from build123d import *

# Parameters (mm, degrees)
PAD_DEPTH       = 4.5
PAD001_DEPTH    = 140
SKETCH002_R     = 20
PAD002_DEPTH    = 17
SKETCH003_R     = 15.5
POCKET_DEPTH    = 17
POCKET001_DEPTH = 140
FILLET_R        = 2
CHAMFER_SIZE    = 2
SKETCH005_R     = 4.5
SKETCH005_R_2   = 1.45
POCKET002_DEPTH = 5


with BuildPart() as part:
    # Sketch → Pad (new body)
    with BuildSketch(Plane.XZ):
        with BuildLine():
            ThreePointArc((14.282857, 14), (-20, 0), (14.282857, -14))
            Line((14.282857, -14), (125.717143, -14))
            ThreePointArc((125.717143, -14), (160, 0), (125.717143, 14))
            Line((14.282857, 14), (125.717143, 14))
        make_face()
    extrude(amount=PAD_DEPTH)

    # Sketch001 → Pad001 (join)
    with BuildSketch(Plane.YZ):
        Polygon((0, 8.637), (10.293176, 0), (0, -8.637), (0, -14), (16.68455, 0), (0, 14), align=None)
    extrude(amount=PAD001_DEPTH)

    # Sketch002 (on Face4 of Pad001) → Pad002 (join)
    with BuildSketch(Plane(origin=(0, 0, 0), x_dir=(1, 0, 0), z_dir=(0, 1, 0))):
        Circle(SKETCH002_R)
        with Locations((140, 0)):
            Circle(SKETCH002_R)
    extrude(amount=PAD002_DEPTH)

    # Sketch003 (on Face9 of Pad002) → Pocket (cut)
    with BuildSketch(Plane(origin=(0, 17, 0), x_dir=(1, 0, 0), z_dir=(0, 1, 0))):
        Circle(SKETCH003_R)
        with Locations((140, 0)):
            Circle(SKETCH003_R)
    extrude(amount=-POCKET_DEPTH, mode=Mode.SUBTRACT)

    # Sketch004 → Pocket001 (cut)
    with BuildSketch(Plane.YZ):
        Polygon((0, 8.635), (0, -8.635), (10.290792, 0), align=None)
    extrude(amount=POCKET001_DEPTH, mode=Mode.SUBTRACT)

    # Fillet
    fillet_edges = [part.edges().sort_by_distance(p)[0] for p in [
        (120, 17, 0),
        (124.5, 17, 0),
        (-20, 17, 0),
        (-15.5, 17, 0),
    ]]
    fillet(fillet_edges, radius=FILLET_R)

    # Chamfer
    chamfer_edges = [part.edges().sort_by_distance(p)[0] for p in [
        (-20, -4.5, 0),
        (70, -4.5, -14),
        (160, -4.5, 0),
        (70, -4.5, 14),
    ]]
    chamfer(chamfer_edges, length=CHAMFER_SIZE)

    # Sketch005 (on Face29 of Chamfer) → Pocket002 (cut)
    with BuildSketch(Plane(origin=(0, 0, 0), x_dir=(1, 0, 0), z_dir=(0, 1, 0))):
        Circle(SKETCH005_R)
        with Locations((13, 0)):
            Circle(SKETCH005_R_2)
        with Locations((-13, 0)):
            Circle(SKETCH005_R_2)
        with Locations((140, 0)):
            Circle(SKETCH005_R)
        with Locations((153, 0)):
            Circle(SKETCH005_R_2)
        with Locations((127, 0)):
            Circle(SKETCH005_R_2)
        with Locations((0, 13)):
            Circle(SKETCH005_R_2)
        with Locations((0, -13)):
            Circle(SKETCH005_R_2)
        with Locations((140, 13)):
            Circle(SKETCH005_R_2)
        with Locations((140, -13)):
            Circle(SKETCH005_R_2)
    extrude(amount=-POCKET002_DEPTH, mode=Mode.SUBTRACT)


solid = part.part
Could you check a few things on this model? Use its own coordinates, in mm. A direction names the side the tool comes from. Give positions to 0.01 mm unless a question says otherwise; leave off trailing zeros. Loops run counter-clockwise (first coordinate to the right, second up) from the corner with the lowest first, then second, coordinate; pieces in that order, holes last. Notation, with made-up numbers: M 53.5,23.5 L 69.5,23.5 A27 cw 69.5,51.5 Z; hole C 72.25,39.25 d9. An arc over 180 degrees is marked long. Answer as a JSON object with one key per item and string values.
Q1. For faces 3 (the cylindrical face through (141.339, -2.218, -12.445)), 4 (the cylindrical face through (-15.485, 7.605, -0.682)), 5 (the flat face through (17.18, 5.07, -4.38)), which set-ups out of +Z, -Z, +X, -X, +Y, -Y let a thin tool reach every point of the face, with its end or its side?
Values found:
{"face 3": "+Y, -Y", "face 4": "+Y", "face 5": "none"}
Q2. If I drill on probe 1 along X at (y, z) = (7, 0); probe 2 along X at (y, z) = (14.5, 13); probe 3 along X at (y, z) = (-3.45, -13), over which ranges is the centre line in solid material (lowest first)? Write a range as [from, to].
Values found:
{"probe 1": "x = [-20, -15.5], [155.5, 160]", "probe 2": "x = [-15.2, -8.44], [8.44, 15.2], [124.8, 131.56], [148.44, 155.2]", "probe 3": "x = [-13.92, -1.45], [1.45, 138.55], [141.45, 153.92]"}
Q3. If we mould it in two halves opening along X, with no side actions, what happens to faces 1 (the flat face through (69, -4.5, 0)), 2 (the cylindrical face through (154.318, 7.605, 5.937))? For each: pulls with the +X half, pulls with the -X half, needs draft (parallel to the pull), parting line crosses it, or undercut.
Values found:
{"face 1": "needs draft", "face 2": "undercut"}
Q4. Suppose I cut it at A-A, the plane x = 37. List the corners of the cut face in (y, z) for me, plus the area to 3 significant figures.
Values found:
{"outline": "M -4.5,-12 L -2.5,-14 L 0,-14 L 16.68,0 L 0,14 L -2.5,14 L -4.5,12 Z; hole M 0,-8.64 L 10.29,0 L 0,8.64 Z", "area": "267 mm²"}
Q5. For P1, Ø4, axis at x = 0, z = 13, coming from the +Y side; P2, Ø1.5, axis at x = 85, z = 12.5, coming from the +Y side; P3, Ø2, axis at x = 124, y = 3, coming from the -Z side, each with a flat end and sliding along its axis, tell me the tip position at first contact or that it passes through.
Values found:
{"P1": "stops at y = 0", "P2": "stops at y = 2.68", "P3": "stops at z = -13.23"}
